from build123d import *

# Parameters (mm, degrees)
SKETCH1_R               = 13.6
BOSS_EXTRUDE1_DEPTH     = 50.7
CUT_EXTRUDE1_DEPTH      = 55.225547485
SKETCH3_R               = 14
SKETCH3_R_2             = 13.6
BOSS_EXTRUDE2_DEPTH     = 47.7
SKETCH4_R               = 14
BOSS_EXTRUDE3_DEPTH     = 15
BOSS_EXTRUDE4_START     = 2
BOSS_EXTRUDE4_DEPTH     = 2
SKETCH6_R               = 1.5
CUT_EXTRUDE2_DEPTH      = 7
SKETCH7_R               = 5.4
BOSS_EXTRUDE5_DEPTH     = 3
SKETCH8_R               = 4
CUT_EXTRUDE3_DEPTH      = 1.5
SKETCH9_R               = 1.7
CUT_EXTRUDE4_DEPTH      = 0.5
CUT_EXTRUDE5_START      = 1.25
SKETCH12_R              = 4.570841128
SKETCH12_R_2            = 4
CUT_EXTRUDE5_DEPTH      = 1.25
FILLET1_R               = 0.5
CHAMFER1_SIZE           = 0.5
CUT_EXTRUDE6_REACH      = 75.756
CUT_EXTRUDE6_END_RADIUS = 12.956768024
SKETCH13_W              = 1.739955734
SKETCH13_H              = 3.306373614
CUT_EXTRUDE7_DEPTH      = 0.5
CUT_EXTRUDE8_DEPTH      = 3.306373613
BOSS_EXTRUDE7_DEPTH     = 3.306373613
SKETCH17_W              = 10.414574722
SKETCH17_H              = 2.75
BOSS_EXTRUDE8_DEPTH     = 4.85
SKETCH18_W              = 9.614574722
SKETCH18_H              = 1.95
CUT_EXTRUDE10_DEPTH     = 4.85
SKETCH20_R              = 0.7
BOSS_EXTRUDE9_DEPTH     = 4.85
SCALE1_SCALE            = 0.25
SKETCH21_R              = 0.348695204
BOSS_EXTRUDE10_DEPTH    = 3


with BuildPart() as part:
    # Sketch1 → Boss-Extrude1 (new body)
    with BuildSketch(Plane(origin=(0, 0, 0), x_dir=(0, 0, -1), z_dir=(1, 0, 0))):
        Circle(SKETCH1_R)
    extrude(amount=-BOSS_EXTRUDE1_DEPTH)

    # Sketch2 → Cut-Extrude1 (cut, through all)
    with BuildSketch(Plane(origin=(0, 0, 0), x_dir=(0, 0, -1), z_dir=(1, 0, 0))):
        with BuildLine():
            Line((-1.476652596, 12.872347678), (-1.476652596, 14.372812182))
            Line((-1.476652596, 14.372812182), (1.476652596, 14.372812182))
            Line((1.476652596, 14.372812182), (1.476652596, 12.872347678))
            ThreePointArc((1.476652596, 12.872347678), (0, 12.956768024), (-1.476652596, 12.872347678))
        make_face()
        with BuildLine():
            Line((1.476652596, -12.872347678), (1.476652596, -14.372812182))
            Line((1.476652596, -14.372812182), (-1.476652596, -14.372812182))
            Line((-1.476652596, -14.372812182), (-1.476652596, -12.872347678))
            ThreePointArc((-1.476652596, -12.872347678), (0, -12.956768024), (1.476652596, -12.872347678))
        make_face()
        with BuildLine():
            Line((11.886106393, -5.157355179), (13.185546772, -5.907587431))
            Line((13.185546772, -5.907587431), (11.708894176, -8.465224751))
            Line((11.708894176, -8.465224751), (10.409453797, -7.714992499))
            ThreePointArc((10.409453797, -7.714992499), (11.220890259, -6.478384012), (11.886106393, -5.157355179))
        make_face()
        with BuildLine():
            Line((-11.886106393, 5.157355179), (-13.185546772, 5.907587431))
            Line((-13.185546772, 5.907587431), (-11.708894176, 8.465224751))
            Line((-11.708894176, 8.465224751), (-10.409453797, 7.714992499))
            ThreePointArc((-10.409453797, 7.714992499), (-11.220890259, 6.478384012), (-11.886106393, 5.157355179))
        make_face()
    extrude(amount=-CUT_EXTRUDE1_DEPTH, mode=Mode.SUBTRACT)



with BuildPart() as body_2:
    # Sketch3 → Boss-Extrude2 (new body)
    with BuildSketch(Plane(origin=(-1, 0, 0), x_dir=(0, 0, -1), z_dir=(1, 0, 0))):
        Circle(SKETCH3_R)
        Circle(SKETCH3_R_2, mode=Mode.SUBTRACT)
    extrude(amount=-BOSS_EXTRUDE2_DEPTH)


with BuildPart() as body_3:
    # Sketch4 → Boss-Extrude3 (new body)
    with BuildSketch(Plane.ZY.offset(50.7)):
        Circle(SKETCH4_R)
    extrude(amount=BOSS_EXTRUDE3_DEPTH)


with BuildPart() as part_1:
    add(part.part)

    add(body_2.part)  # Boss-Extrude4 merges body 2

    add(body_3.part)  # Boss-Extrude4 merges body 3
    # Sketch5 → Boss-Extrude4 (add)
    with BuildSketch(Plane(origin=(-50.7, 0, 0), x_dir=(0, 0, -1), z_dir=(1, 0, 0)).offset(BOSS_EXTRUDE4_START)):
        with BuildLine():
            Line((1.476652596, 13.519596781), (1.498368075, 13.71841438))
            ThreePointArc((1.498368075, 13.71841438), (11.951150572, 6.9), (12.629679391, -5.561582373))
            Line((12.629679391, -5.561582373), (12.446640559, -5.48097973))
            ThreePointArc((12.446640559, -5.48097973), (11.777945491, 6.8), (1.476652596, 13.519596781))
        make_face()
        with BuildLine():
            Line((-1.476652596, 13.519596781), (-1.498368075, 13.71841438))
            ThreePointArc((-1.498368075, 13.71841438), (-6.9, 11.951150572), (-11.131311316, 8.156832007))
            Line((-11.131311316, 8.156832007), (-10.969987963, 8.038617051))
            ThreePointArc((-10.969987963, 8.038617051), (-6.8, 11.777945491), (-1.476652596, 13.519596781))
        make_face()
        with BuildLine():
            Line((10.969987963, -8.038617051), (11.131311316, -8.156832007))
            ThreePointArc((11.131311316, -8.156832007), (6.9, -11.951150572), (1.498368075, -13.71841438))
            Line((1.498368075, -13.71841438), (1.476652596, -13.519596781))
            ThreePointArc((1.476652596, -13.519596781), (6.8, -11.777945491), (10.969987963, -8.038617051))
        make_face()
        with BuildLine():
            Line((-1.476652596, -13.519596781), (-1.498368075, -13.71841438))
            ThreePointArc((-1.498368075, -13.71841438), (-11.951150572, -6.9), (-12.629679391, 5.561582373))
            Line((-12.629679391, 5.561582373), (-12.446640559, 5.48097973))
            ThreePointArc((-12.446640559, 5.48097973), (-11.777945491, -6.8), (-1.476652596, -13.519596781))
        make_face()
    extrude(amount=-BOSS_EXTRUDE4_DEPTH)

    # Sketch6 → Cut-Extrude2 (cut)
    with BuildSketch(Plane(origin=(0, 0, 0), x_dir=(0, 0, -1), z_dir=(1, 0, 0))):
        with Locations((-5, -8.660254038)):
            Circle(SKETCH6_R)
        with Locations((5, 8.660254038)):
            Circle(SKETCH6_R)
        with Locations((-7.794228634, 4.5)):
            Circle(SKETCH6_R)
        with Locations((7.794228634, -4.5)):
            Circle(SKETCH6_R)
    extrude(amount=-CUT_EXTRUDE2_DEPTH, mode=Mode.SUBTRACT)

    # Sketch7 → Boss-Extrude5 (add)
    with BuildSketch(Plane(origin=(0, 0, 0), x_dir=(0, 0, -1), z_dir=(1, 0, 0))):
        Circle(SKETCH7_R)
    extrude(amount=BOSS_EXTRUDE5_DEPTH)

    # Sketch8 → Cut-Extrude3 (cut)
    with BuildSketch(Plane(origin=(3, 0, 0), x_dir=(0, 0, -1), z_dir=(1, 0, 0))):
        Circle(SKETCH8_R)
    extrude(amount=-CUT_EXTRUDE3_DEPTH, mode=Mode.SUBTRACT)

    # Sketch9 → Cut-Extrude4 (cut)
    with BuildSketch(Plane(origin=(1.5, 0, 0), x_dir=(0, 0, -1), z_dir=(1, 0, 0))):
        Circle(SKETCH9_R)
    extrude(amount=-CUT_EXTRUDE4_DEPTH, mode=Mode.SUBTRACT)

    # Sketch12 → Cut-Extrude5 (cut)
    with BuildSketch(Plane(origin=(1.5, 0, 0), x_dir=(0, 0, -1), z_dir=(1, 0, 0)).offset(CUT_EXTRUDE5_START)):
        Circle(SKETCH12_R)
        Circle(SKETCH12_R_2, mode=Mode.SUBTRACT)
    extrude(amount=-CUT_EXTRUDE5_DEPTH, mode=Mode.SUBTRACT)

    # Fillet1
    fillet1_edges = [part_1.edges().sort_by_distance(p)[0] for p in [
        (0, 0, 5.4),
        (3, 0, 5.4),
    ]]
    fillet(fillet1_edges, radius=FILLET1_R)

    # Chamfer1
    chamfer1_edges = [part_1.edges().sort_by_distance(p)[0] for p in [
        (-65.7, 0, -14),
        (0, 11.777945491, 6.8),
        (0, -6.8, 11.777945491),
        (0, -11.777945491, -6.8),
        (0, 6.8, -11.777945491),
    ]]
    chamfer(chamfer1_edges, length=CHAMFER1_SIZE)

    # Cut-Extrude6: up to this cylinder (the profile starts outside it)
    cut_extrude6_end = Plane(origin=(-57.95, 0, 0), z_dir=(1, 0, 0)) * Cylinder(CUT_EXTRUDE6_END_RADIUS, 178.425536047, mode=Mode.PRIVATE)
    # Sketch13 → Cut-Extrude6 (cut, up to the surface)
    with BuildSketch(Plane(origin=(0, 12.124355653, 7), x_dir=(1, 0, 0), z_dir=(0, 0.866025403784438, 0.500000000000001)), mode=Mode.PRIVATE) as cut_extrude6_sk1:
        with Locations((-57.95, 0)):
            Rectangle(SKETCH13_W, SKETCH13_H)
    cut_extrude6_tool1 = extrude(cut_extrude6_sk1.sketch, amount=-CUT_EXTRUDE6_REACH, mode=Mode.PRIVATE) - cut_extrude6_end
    cut_extrude6 = cut_extrude6_tool1.solids().sort_by_distance((-57.95, 12.124356, 7))[0]
    add(cut_extrude6, mode=Mode.SUBTRACT)

    # Sketch14 → Cut-Extrude7 (cut)
    with BuildSketch(Plane(origin=(-58.819977867, 0, 0), x_dir=(0, 0, -1), z_dir=(1, 0, 0))):
        with BuildLine():
            Line((-5.256527567, 12.41094643), (-8.11993111, 10.757759624))
            Line((-8.11993111, 10.757759624), (-7.857135823, 10.302584835))
            ThreePointArc((-7.857135823, 10.302584835), (-6.478384012, 11.220890259), (-4.99373228, 11.955771641))
            Line((-4.99373228, 11.955771641), (-5.256527567, 12.41094643))
        make_face()
    cut_extrude7 = extrude(amount=-CUT_EXTRUDE7_DEPTH, mode=Mode.SUBTRACT)

    # Sketch15 → Cut-Extrude8 (cut)
    with BuildSketch(Plane(origin=(0, 0.826593403, -1.431701772), x_dir=(1, 0, 0), z_dir=(0, -0.5000000000000011, 0.8660254037844379))):
        Polygon((-58.819977867, 13.902049251), (-59.319977867, 12.850868103), (-58.819977867, 12.850868103), align=None)
    cut_extrude8 = extrude(amount=CUT_EXTRUDE8_DEPTH, mode=Mode.SUBTRACT)

    # Sketch16 → Boss-Extrude7 (add)
    with BuildSketch(Plane(origin=(0, 0.826593403, -1.431701772), x_dir=(1, 0, 0), z_dir=(0, -0.5000000000000011, 0.8660254037844379))):
        Polygon((-59.069977867, 13.376458677), (-59.319977867, 12.850868103), (-59.319977867, 13.376458677), align=None)
    boss_extrude7 = extrude(amount=BOSS_EXTRUDE7_DEPTH)

    # Mirror1: Cut-Extrude6, Cut-Extrude7, Cut-Extrude8, Boss-Extrude7 across plane
    add(cut_extrude6.mirror(Plane(origin=(0, 0, 0), x_dir=(0, -0.500000000000001, 0.866025403784438), z_dir=(0, 0.866025403784438, 0.500000000000001))), mode=Mode.SUBTRACT)
    add(cut_extrude7.mirror(Plane(origin=(0, 0, 0), x_dir=(0, -0.500000000000001, 0.866025403784438), z_dir=(0, 0.866025403784438, 0.500000000000001))), mode=Mode.SUBTRACT)
    add(cut_extrude8.mirror(Plane(origin=(0, 0, 0), x_dir=(0, -0.500000000000001, 0.866025403784438), z_dir=(0, 0.866025403784438, 0.500000000000001))), mode=Mode.SUBTRACT)
    add(boss_extrude7.mirror(Plane(origin=(0, 0, 0), x_dir=(0, -0.500000000000001, 0.866025403784438), z_dir=(0, 0.866025403784438, 0.500000000000001))))


with BuildPart() as body_2_2:
    # Sketch17 → Boss-Extrude8 (new body)
    with BuildSketch(Plane.ZY.offset(65.7)):
        with Locations((0, 8.736671017)):
            Rectangle(SKETCH17_W, SKETCH17_H)
    extrude(amount=BOSS_EXTRUDE8_DEPTH)

    # Sketch18 → Cut-Extrude10 (cut)
    with BuildSketch(Plane.ZY.offset(70.55)):
        with Locations((0, 8.736671017)):
            Rectangle(SKETCH18_W, SKETCH18_H)
    extrude(amount=-CUT_EXTRUDE10_DEPTH, mode=Mode.SUBTRACT)


    add(part_1.part)  # Boss-Extrude9 merges part
    # Sketch20 → Boss-Extrude9 (add)
    with BuildSketch(Plane.ZY.offset(65.7)):
        with Locations(Location((0, 8.736671017, 0), (0, 0, 180))):
            Circle(SKETCH20_R)
        with Locations(Location((1.8, 8.736671017, 0), (0, 0, 180))):
            Circle(SKETCH20_R)
        with Locations(Location((3.6, 8.736671017, 0), (0, 0, 180))):
            Circle(SKETCH20_R)
        with Locations(Location((-1.8, 8.736671017, 0), (0, 0, 180))):
            Circle(SKETCH20_R)
        with Locations(Location((-3.6, 8.736671017, 0), (0, 0, 180))):
            Circle(SKETCH20_R)
    extrude(amount=BOSS_EXTRUDE9_DEPTH)


with BuildPart() as body_2_2_1:
    # Scale1: scaled about (-32.994808114, 0.01862081, 0)
    add(body_2_2.part.scale(SCALE1_SCALE).moved(Location((-24.746106086, 0.013965608, 0))))

    # Sketch21 → Boss-Extrude10 (add)
    with BuildSketch(Plane(origin=(-24.496106086, 0, 0), x_dir=(0, 0, -1), z_dir=(1, 0, 0))):
        Circle(SKETCH21_R)
    extrude(amount=BOSS_EXTRUDE10_DEPTH)


solid = body_2_2_1.part
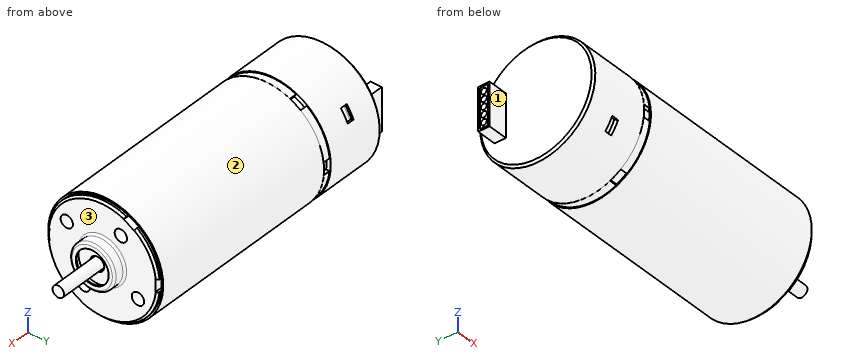
Check sheet for the modelled part. Datum: model origin and axes. Units: mm. Face numbers are marked on the shaded views. A direction names the side the tool comes from. Give positions to 0.01 mm unless a question says otherwise; leave off trailing zeros. Loops run counter-clockwise (first coordinate to the right, second up) from the corner with the lowest first, then second, coordinate; pieces in that order, holes last. Notation, with made-up numbers: M 84.25,-27.5 L 119.25,-27.5 A18 cw 119.25,-22.5 Z; hole C 15.25,-13.75 d2. An arc over 180 degrees is marked long. Return JSON: item names as keys, results as strings. Group by question number.
1. Go/stop test with flat-tipped pins: pin 1 (0.6 mm diameter, centred on x = -42, z = 0, fed in from -Y); pin 2 (0.6 mm diameter, centred on y = -1, z = -2, fed in from +X); pin 3 (0.5 mm diameter, centred on y = -2.5, z = -1.5, fed in from -X). Record where each tip stops, or that it passes through.
2. Cross-section at B-B on x = -40.75. Record the boundary of the cut face in (y, z).
3. Tool access check on the marked faces 1, 2 and 3. Record the directions out of +Z, -Z, +X, -X, +Y, -Y that give a thin tool (end or side, any length) a straight path to the whole face; none if there is none.
4. Thickness scan on L1, parallel to Y at x = -24.15, z = 0; L2, parallel to X at y = -0.5, z = 1.5; L3, parallel to X at y = 2.25, z = 0.5. Record the ranges inside material, lowest first.
5. Cross-section at A-A on x = -25.75. State how many separate pieces and enclosed holes the cut face has, plus the area to 3 significant figures.
Return value:
{
 "1": {"pin 1": "y = 1.85", "pin 2": "x = -24.75", "pin 3": "x = -41.17"},
 "2": {"outline": "C 0.01,0 d7"},
 "3": {"face 1": "+Z, -Z, -X, -Y", "face 2": "+X, -X", "face 3": "+X"},
 "4": {"L1": "-1.34 to -1.13, -0.35 to 0.35, 1.16 to 1.36", "L2": "-41.17 to -24.75", "L3": "-42.38 to -24.75"},
 "5": {"separate pieces": "1", "enclosed holes": "8", "area": "36.2 mm^2"}
}
